The model under review builds one solid part; all positions refer to its coordinate system, in mm. A direction names the side the tool comes from. Give positions to 0.01 mm unless a question says otherwise; leave off trailing zeros. Order: outer loops, then holes, each group sorted by start corner. A loop starts at its lowest first (then second) coordinate and runs counter-clockwise, first axis right, second up. Notation, with made-up numbers: (69.25, 68) - (97.25, 68) arc R22 ccw to (97.25, 94) - close; hole circle Ø4 at (-2.75, -10.5). An arc over 180 degrees is marked (long way). Put each result on its own line as item: value.
```python
from build123d import *

# Parameters (mm, degrees)
BOSS_EXTRUDE1_DEPTH = 3
SKETCH2_R           = 4.975
SKETCH2_R_2         = 3.975
EXTRUDE_THIN1_DEPTH = 4


with BuildPart() as part:
    # Sketch1 → Boss-Extrude1 (new body)
    with BuildSketch(Plane.XY):
        with BuildLine():
            Line((-28.620254205, 6.475802165), (0.164228554, 3.985109024))
            ThreePointArc((0.164228554, 3.985109024), (3.819400968, 0), (0.164228554, -3.985109024))
            Line((0.164228554, -3.985109024), (-28.620254205, -6.475802165))
            ThreePointArc((-28.620254205, -6.475802165), (-35.680599032, 0), (-28.620254205, 6.475802165))
        make_face()
    extrude(amount=BOSS_EXTRUDE1_DEPTH)

    # Sketch2 → Extrude-Thin1 (add)
    with BuildSketch(Plane.XY.offset(3)):
        with Locations((-29.180599032, 0)):
            Circle(SKETCH2_R)
        with Locations((-29.180599032, 0)):
            Circle(SKETCH2_R_2, mode=Mode.SUBTRACT)
    extrude(amount=EXTRUDE_THIN1_DEPTH)


solid = part.part
```
(1) Take a section at C-C, the plane x = -14. Write out the cut boundary in (y, z).
The answers:
outline: (-5.21, 0) - (5.21, 0) - (5.21, 3) - (-5.21, 3) - close
(2) The part is to be moulded in two halves that separate along Y. For faces 3 (the flat face through (-16, 0, 3)), 4 (the cylindrical face through (3.82, 0.08, 1.48)), 5 (the flat face through (-29, 0, 3)), say which applies: pulls with the +Y half, pulls with the -Y half, needs draft (parallel to the pull), parting line crosses it, or undercut.
The answers:
face 3: needs draft
face 4: parting line crosses it
face 5: undercut
(3) Take a section at D-D, the plane y = -2.75. Write out the cut boundary in (x, z), then the cut area to 3 significant figures.
The answers:
outline: (-35.07, 0) - (2.72, 0) - (2.72, 3) - (-25.03, 3) - (-25.03, 7) - (-26.31, 7) - (-26.31, 3) - (-32.05, 3) - (-32.05, 7) - (-33.33, 7) - (-33.33, 3) - (-35.07, 3) - close
area: 124 mm^2
(4) Clearance check with flat-ended pins moving along their axes: pin 1 Ø3 at (y, z) = (-2.5, 2) entering from +X; pin 2 Ø1 at (x, y) = (-7, -0.5) entering from -Z; pin 3 Ø1 at (y, z) = (0, 4.5) entering from +X; pin 4 Ø1 at (y, z) = (2, 5) entering from -X. State where each tip first meets the part, or that it passes through.
The answers:
pin 1: x = 3.69
pin 2: z = 0
pin 3: x = -24.21
pin 4: x = -33.92
(5) Wall thickness on L1, parallel to Z at x = -1, y = 1.25; L2, parallel to X at y = -1, z = 3.75; L3, parallel to Y at x = -31, z = 6.5: over which ranges is each line inside the solid? List them lowest first.
The answers:
L1: 0 to 3
L2: -34.05 to -33.03, -25.33 to -24.31
L3: -4.63 to -3.53, 3.53 to 4.63
(6) For faces 1 (the cylindrical face through (-24.435, 1.494, 4.972)), 2 (the flat face through (-14.027, -5.213, 1.479)), list the 3-axis set-ups (+Z, -Z, +X, -X, +Y, -Y) from which the entire face can be reached by the end or side of a thin tool; tool diameter is ignored.
The answers:
face 1: +Z
face 2: +Z, -Z, +X, -Y
(7) Take a section at B-B, the plane z = 4.5. Write out the cut boundary in (x, y) (3 decimals), then the cut area to 3 significant figures.
The answers:
outline: circle Ø9.95 at (-29.181, 0); hole circle Ø7.95 at (-29.181, 0)
area: 28.1 mm^2
(8) Take a section at A-A, the plane y = 0. Write out the cut boundary in (x, z).
The answers:
outline: (-35.68, 0) - (3.82, 0) - (3.82, 3) - (-24.21, 3) - (-24.21, 7) - (-25.21, 7) - (-25.21, 3) - (-33.16, 3) - (-33.16, 7) - (-34.16, 7) - (-34.16, 3) - (-35.68, 3) - close
